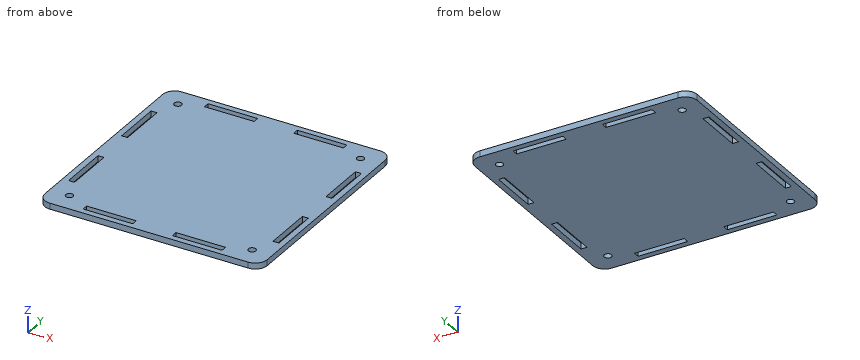
from build123d import *

# Parameters (mm, degrees)
SKETCH_R      = 1.85
SKETCH_W      = 25
SKETCH_H      = 3
SKETCH_W_2    = 3
SKETCH_H_2    = 25
EXTRUDE_DEPTH = 3


with BuildPart() as part:
    # Sketch → Extrude (new body)
    with BuildSketch(Plane.XY):
        with BuildLine():
            ThreePointArc((0, 106), (-4.242641, 104.242641), (-6, 100))
            Line((-6, 100), (-6, 0))
            ThreePointArc((-6, 0), (-4.242641, -4.242641), (0, -6))
            Line((0, -6), (100, -6))
            ThreePointArc((100, -6), (104.242641, -4.242641), (106, 0))
            Line((106, 0), (106, 100))
            ThreePointArc((106, 100), (104.242641, 104.242641), (100, 106))
            Line((0, 106), (100, 106))
        make_face()
        with Locations((4, 96)):
            Circle(SKETCH_R, mode=Mode.SUBTRACT)
        with Locations((96, 96)):
            Circle(SKETCH_R, mode=Mode.SUBTRACT)
        with Locations((96, 4)):
            Circle(SKETCH_R, mode=Mode.SUBTRACT)
        with Locations((4, 4)):
            Circle(SKETCH_R, mode=Mode.SUBTRACT)
        with Locations((27.5, 101.5)):
            Rectangle(SKETCH_W, SKETCH_H, mode=Mode.SUBTRACT)
        with Locations((72.5, 101.5)):
            Rectangle(SKETCH_W, SKETCH_H, mode=Mode.SUBTRACT)
        with Locations((101.5, 72.5)):
            Rectangle(SKETCH_W_2, SKETCH_H_2, mode=Mode.SUBTRACT)
        with Locations((101.5, 27.5)):
            Rectangle(SKETCH_W_2, SKETCH_H_2, mode=Mode.SUBTRACT)
        with Locations((72.5, -1.5)):
            Rectangle(SKETCH_W, SKETCH_H, mode=Mode.SUBTRACT)
        with Locations((27.5, -1.5)):
            Rectangle(SKETCH_W, SKETCH_H, mode=Mode.SUBTRACT)
        with Locations((-1.5, 27.5)):
            Rectangle(SKETCH_W_2, SKETCH_H_2, mode=Mode.SUBTRACT)
        with Locations((-1.5, 72.5)):
            Rectangle(SKETCH_W_2, SKETCH_H_2, mode=Mode.SUBTRACT)
    extrude(amount=EXTRUDE_DEPTH)


solid = part.part
The model under review builds one solid part; all positions refer to its coordinate system, in mm. Coordinates: 2 decimals unless noted, no trailing zeros. Loops run counter-clockwise (first coordinate to the right, second up) from the corner with the lowest first, then second, coordinate; pieces in that order, holes last. Notation, with made-up numbers: M 22.5,86.5 L 45.5,86.5 A14 cw 45.5,96.5 Z; hole C -38,13.5 d4. An arc over 180 degrees is marked long. Put each result on its own line as item: value. Start each with the question number.
Q1. Add section A-A (y = 80). Write out the cut boundary in (x, z), and give its area (3 significant figures).
Q2. Add section C-C (z = 0.9). Count the separate pieces of the cut face and the enclosed holes in it, and give its area (3 significant figures).
Q3. Add section B-B (x = 96). Write out the cut boundary in (y, z), and give its area (3 significant figures).
Q4. Clearance check with flat-ended pins moving along their axes: pin 1 (0.9 mm diameter, centred on y = 101.5, z = 1, fed in from -X); pin 2 (0.9 mm diameter, centred on x = 101.5, z = 1, fed in from -Y); pin 3 (3 mm diameter, centred on x = 96, y = 96, fed in from +Z). State where each tip first meets the part, or that it passes through.
Q5. Wall thickness on line 1 (X direction, y = 73, z = 2.95); line 2 (X direction, y = 96, z = 2.2): over which ranges is each line inside the solid? List them lowest first.
Answers:
1. outline: M -6,0 L -3,0 L -3,3 L -6,3 Z; M 0,0 L 100,0 L 100,3 L 0,3 Z; M 103,0 L 106,0 L 106,3 L 103,3 Z
1. area: 318 mm^2
2. separate pieces: 1
2. enclosed holes: 12
2. area: 11,900 mm^2
3. outline: M -6,0 L 2.15,0 L 2.15,3 L -6,3 Z; M 5.85,0 L 94.15,0 L 94.15,3 L 5.85,3 Z; M 97.85,0 L 106,0 L 106,3 L 97.85,3 Z
3. area: 314 mm^2
4. pin 1: stops at x = -5.91
4. pin 2: stops at y = -5.91
4. pin 3: passes through
5. line 1: x = -6 to -3, 0 to 100, 103 to 106
5. line 2: x = -6 to 2.15, 5.85 to 94.15, 97.85 to 106
